The listing builds one solid part. Answer for the finished solid, in the listing's coordinates (mm). A direction names the side the tool comes from. Coordinates: 2 decimals unless noted, no trailing zeros. Order: outer loops, then holes, each group sorted by start corner. A loop starts at its lowest first (then second) coordinate and runs counter-clockwise, first axis right, second up. Notation, with made-up numbers: (-3, 74.5) - (13, 74.5) arc R32 cw to (13, 112.5) - close; hole circle Ø1 at (87.25, 50). An arc over 180 degrees is marked (long way). Use a Markdown table: item, result. Add a question column.
Item 1: The part is cut by section A-A, the plane z = 62. State how many separate pieces and enclosed holes the cut face has, then the cut area to 3 significant figures.
Item 2: Find the intervals of material crossed by line 1 along X through (y, z) = (-29.5, 34); line 2 along Y through (x, z) = (0, 8); line 3 along Y through (x, z) = (0, 41), in increasing order.
Item 3: The part is cut by section B-B, the plane x = 0. Give the vertices of the cut face in (y, z), then the cut area to 3 significant figures.
Item 4: For faces 5 (the cylindrical face through (13.887, -10.648, 4.93)), 6 (the cylindrical face through (23.334, 20.721, 16.661)), 7 (the flat face through (32.5, 0, 33)), determine the directions among +Z, -Z, +X, -X, +Y, -Y from which every point of the face is accessible in a straight line to the end or side of a thin tool.
Item 5: Flat-ended cylindrical pins translate along their axes: P1, Ø10, axis at y = 28, z = 36.5, coming from the +X side; P2, Ø1.5, axis at y = 1, z = 34.5, coming from the -X side; P3, Ø1.5, axis at x = 19.5, y = -22, coming from the -Z side; P4, Ø20, axis at x = 31, y = -34, coming from the +Z side. Find the tip coordinate at first contact, or state that the pin passes through.
Item 6: The part is cut by section C-C, the plane z = 33.5. Give the vertices of the cut face in (x, y), then the cut area to 3 significant figures.
Item 7: The mould has two halves that part along Y. Classify faces 1 (the flat face through (-32, 32, 60)), 2 (the flat face through (-41, -18, 70)), 3 (the cylindrical face through (46.187, -19.15, 34.51)), 4 (the flat face through (36.92, -25.85, 65.07)): released by +Y, released by -Y, zero draft, split by the parting line, or undercut.
from build123d import *

# Parameters (mm, degrees)
CROQUIS1_R              = 50
CROQUIS1_R_2            = 15.5
SALIENTE_EXTRUIR1_DEPTH = 70
CROQUIS2_R              = 40
CORTAR_EXTRUIR1_DEPTH   = 32
CROQUIS3_R              = 17.5
CORTAR_EXTRUIR2_DEPTH   = 10
CROQUIS4_R              = 40
CROQUIS4_R_2            = 15.5
CORTAR_EXTRUIR3_DEPTH   = 10
CROQUIS5_R              = 2
CORTAR_EXTRUIR4_DEPTH   = 83.24354078
CROQUIS6_R              = 5
CORTAR_EXTRUIR5_DEPTH   = 5
CORTAR_EXTRUIR6_DEPTH   = 10


with BuildPart() as part:
    # Croquis1 → Saliente-Extruir1 (new body)
    with BuildSketch(Plane.XY):
        Circle(CROQUIS1_R)
        Circle(CROQUIS1_R_2, mode=Mode.SUBTRACT)
    extrude(amount=SALIENTE_EXTRUIR1_DEPTH)

    # Croquis2 → Cortar-Extruir1 (cut)
    with BuildSketch(Plane.XY.offset(70)):
        Circle(CROQUIS2_R)
    extrude(amount=-CORTAR_EXTRUIR1_DEPTH, mode=Mode.SUBTRACT)

    # Croquis3 → Cortar-Extruir2 (cut)
    with BuildSketch(Plane(origin=(0, 0, 0), x_dir=(-1, 0, 0), z_dir=(0, 0, -1))):
        Circle(CROQUIS3_R)
    extrude(amount=-CORTAR_EXTRUIR2_DEPTH, mode=Mode.SUBTRACT)

    # Croquis4 → Cortar-Extruir3 (cut)
    # profile 1 of 2: a face of its own
    with BuildSketch(Plane.XY.offset(38)):
        Circle(CROQUIS4_R)
        with BuildLine():
            Line((-2.5, 27.386127875), (-2.5, 32.5))
            Line((-2.5, 32.5), (2.5, 32.5))
            Line((2.5, 32.5), (2.5, 27.386127875))
            ThreePointArc((2.5, 27.386127875), (19.445436483, 19.445436483), (27.386127875, 2.5))
            Line((27.386127875, 2.5), (32.5, 2.5))
            Line((32.5, 2.5), (32.5, -2.5))
            Line((32.5, -2.5), (27.386127875, -2.5))
            ThreePointArc((27.386127875, -2.5), (19.445436483, -19.445436483), (2.5, -27.386127875))
            Line((2.5, -27.386127875), (2.5, -32.5))
            Line((2.5, -32.5), (-2.5, -32.5))
            Line((-2.5, -32.5), (-2.5, -27.386127875))
            ThreePointArc((-2.5, -27.386127875), (-19.445436483, -19.445436483), (-27.386127875, -2.5))
            Line((-27.386127875, -2.5), (-32.5, -2.5))
            Line((-32.5, -2.5), (-32.5, 2.5))
            Line((-32.5, 2.5), (-27.386127875, 2.5))
            ThreePointArc((-27.386127875, 2.5), (-19.445436483, 19.445436483), (-2.5, 27.386127875))
        make_face(mode=Mode.SUBTRACT)
    # profile 2 of 2: a face of its own
    with BuildSketch(Plane.XY.offset(38)):
        with BuildLine():
            Line((-2.5, 22.5), (-2.5, 27.386127875))
            ThreePointArc((-2.5, 27.386127875), (-19.445436483, 19.445436483), (-27.386127875, 2.5))
            Line((-27.386127875, 2.5), (-22.5, 2.5))
            Line((-22.5, 2.5), (-22.5, -2.5))
            Line((-22.5, -2.5), (-27.386127875, -2.5))
            ThreePointArc((-27.386127875, -2.5), (-19.445436483, -19.445436483), (-2.5, -27.386127875))
            Line((-2.5, -27.386127875), (-2.5, -22.5))
            Line((-2.5, -22.5), (2.5, -22.5))
            Line((2.5, -22.5), (2.5, -27.386127875))
            ThreePointArc((2.5, -27.386127875), (19.445436483, -19.445436483), (27.386127875, -2.5))
            Line((27.386127875, -2.5), (22.5, -2.5))
            Line((22.5, -2.5), (22.5, 2.5))
            Line((22.5, 2.5), (27.386127875, 2.5))
            ThreePointArc((27.386127875, 2.5), (19.445436483, 19.445436483), (2.5, 27.386127875))
            Line((2.5, 27.386127875), (2.5, 22.5))
            Line((2.5, 22.5), (-2.5, 22.5))
        make_face()
        with Locations(Location((0, 0, 0), (0, 0, 180))):
            Circle(CROQUIS4_R_2, mode=Mode.SUBTRACT)
    extrude(amount=-CORTAR_EXTRUIR3_DEPTH, mode=Mode.SUBTRACT)

    # Croquis5 → Cortar-Extruir4 (cut, through all)
    with BuildSketch(Plane.XY.offset(28)):
        with Locations((21.486974797, 21.486974797)):
            Circle(CROQUIS5_R)
        with Locations((21.486974797, -21.486974797)):
            Circle(CROQUIS5_R)
        with Locations((-21.486974797, -21.486974797)):
            Circle(CROQUIS5_R)
        with Locations((-21.486974797, 21.486974797)):
            Circle(CROQUIS5_R)
    extrude(amount=-CORTAR_EXTRUIR4_DEPTH, mode=Mode.SUBTRACT)

    # Croquis6 → Cortar-Extruir5 (cut)
    with BuildSketch(Plane(origin=(0, 0, 0), x_dir=(-1, 0, 0), z_dir=(0, 0, -1))):
        with Locations((-21.486974797, 21.486974797)):
            Circle(CROQUIS6_R)
        with Locations((21.486974797, 21.486974797)):
            Circle(CROQUIS6_R)
        with Locations((21.486974797, -21.486974797)):
            Circle(CROQUIS6_R)
        with Locations((-21.486974797, -21.486974797)):
            Circle(CROQUIS6_R)
    extrude(amount=-CORTAR_EXTRUIR5_DEPTH, mode=Mode.SUBTRACT)

    # Croquis7 → Cortar-Extruir6 (cut)
    with BuildSketch(Plane.XY.offset(70)):
        with BuildLine():
            ThreePointArc((-6.945927107, 39.39231012), (-3.48622971, 39.847787924), (0, 40))
            Line((0, 40), (0, 50))
            ThreePointArc((0, 50), (-4.357787137, 49.809734905), (-8.682408883, 49.240387651))
            Line((-8.682408883, 49.240387651), (-6.945927107, 39.39231012))
        make_face()
        with BuildLine():
            Line((0, 50), (0, 40))
            ThreePointArc((0, 40), (3.48622971, 39.847787924), (6.945927107, 39.39231012))
            Line((6.945927107, 39.39231012), (8.682408883, 49.240387651))
            ThreePointArc((8.682408883, 49.240387651), (4.357787137, 49.809734905), (0, 50))
        make_face()
        with BuildLine():
            ThreePointArc((22.943057454, 32.766081772), (28.284271247, 28.284271247), (32.766081772, 22.943057454))
            Line((32.766081772, 22.943057454), (40.957602214, 28.678821818))
            ThreePointArc((40.957602214, 28.678821818), (35.355339059, 35.355339059), (28.678821818, 40.957602214))
            Line((28.678821818, 40.957602214), (22.943057454, 32.766081772))
        make_face()
        with BuildLine():
            ThreePointArc((40, 0), (39.847787924, -3.48622971), (39.39231012, -6.945927107))
            Line((39.39231012, -6.945927107), (49.240387651, -8.682408883))
            ThreePointArc((49.240387651, -8.682408883), (49.809734905, -4.357787137), (50, 0))
            ThreePointArc((50, 0), (49.809734905, 4.357787137), (49.240387651, 8.682408883))
            Line((49.240387651, 8.682408883), (39.39231012, 6.945927107))
            ThreePointArc((39.39231012, 6.945927107), (39.847787924, 3.48622971), (40, 0))
        make_face()
        with BuildLine():
            ThreePointArc((32.766081772, -22.943057454), (28.284271247, -28.284271247), (22.943057454, -32.766081772))
            Line((22.943057454, -32.766081772), (28.678821818, -40.957602214))
            ThreePointArc((28.678821818, -40.957602214), (35.355339059, -35.355339059), (40.957602214, -28.678821818))
            Line((40.957602214, -28.678821818), (32.766081772, -22.943057454))
        make_face()
        with BuildLine():
            ThreePointArc((-32.766081772, 22.943057454), (-28.284271247, 28.284271247), (-22.943057454, 32.766081772))
            Line((-22.943057454, 32.766081772), (-28.678821818, 40.957602214))
            ThreePointArc((-28.678821818, 40.957602214), (-35.355339059, 35.355339059), (-40.957602214, 28.678821818))
            Line((-40.957602214, 28.678821818), (-32.766081772, 22.943057454))
        make_face()
        with BuildLine():
            ThreePointArc((-39.39231012, -6.945927107), (-40, 0), (-39.39231012, 6.945927107))
            Line((-39.39231012, 6.945927107), (-49.240387651, 8.682408883))
            ThreePointArc((-49.240387651, 8.682408883), (-50, 0), (-49.240387651, -8.682408883))
            Line((-49.240387651, -8.682408883), (-39.39231012, -6.945927107))
        make_face()
        with BuildLine():
            ThreePointArc((-22.943057454, -32.766081772), (-28.284271247, -28.284271247), (-32.766081772, -22.943057454))
            Line((-32.766081772, -22.943057454), (-40.957602214, -28.678821818))
            ThreePointArc((-40.957602214, -28.678821818), (-35.355339059, -35.355339059), (-28.678821818, -40.957602214))
            Line((-28.678821818, -40.957602214), (-22.943057454, -32.766081772))
        make_face()
        with BuildLine():
            ThreePointArc((6.945927107, -39.39231012), (0, -40), (-6.945927107, -39.39231012))
            Line((-6.945927107, -39.39231012), (-8.682408883, -49.240387651))
            ThreePointArc((-8.682408883, -49.240387651), (0, -50), (8.682408883, -49.240387651))
            Line((8.682408883, -49.240387651), (6.945927107, -39.39231012))
        make_face()
    extrude(amount=-CORTAR_EXTRUIR6_DEPTH, mode=Mode.SUBTRACT)


solid = part.part
Solution:
| question | item | result |
|---|---|---|
| 1 | separate pieces | 8 |
| 1 | enclosed holes | 0 |
| 1 | area | 1,570 mm2 |
| 2 | line 1 | x = -40.37 to -27.01, -2.5 to 2.5, 27.01 to 40.37 |
| 2 | line 2 | y = -50 to -17.5, 17.5 to 50 |
| 2 | line 3 | y = -50 to -40, 40 to 50 |
| 3 | outline | (-50, 0) - (-17.5, 0) - (-17.5, 10) - (-15.5, 10) - (-15.5, 28) - (-22.5, 28) - (-22.5, 38) - (-32.5, 38) - (-32.5, 28) - (-40, 28) - (-40, 60) - (-50, 60) - close; (15.5, 10) - (17.5, 10) - (17.5, 0) - (50, 0) - (50, 60) - (40, 60) - (40, 28) - (32.5, 28) - (32.5, 38) - (22.5, 38) - (22.5, 28) - (15.5, 28) - close |
| 3 | area | 2,730 mm2 |
| 4 | face 5 | -Z |
| 4 | face 6 | +Z, -Z |
| 4 | face 7 | +Z |
| 5 | P1 | stops at x = 44.4 |
| 5 | P2 | stops at x = -50 |
| 5 | P3 | stops at z = 5 |
| 5 | P4 | stops at z = 70 |
| 6 | outline | circle Ø100 at (0, 0); (-32.5, -2.5) - (-22.5, -2.5) - (-22.5, 2.5) - (-32.5, 2.5) - close; (-2.5, -32.5) - (2.5, -32.5) - (2.5, -22.5) - (-2.5, -22.5) - close; (-2.5, 22.5) - (2.5, 22.5) - (2.5, 32.5) - (-2.5, 32.5) - close; (22.5, -2.5) - (32.5, -2.5) - (32.5, 2.5) - (22.5, 2.5) - close; hole circle Ø80 at (0, 0) |
| 6 | area | 3,030 mm2 |
| 7 | face 1 | undercut |
| 7 | face 2 | zero draft |
| 7 | face 3 | split by the parting line |
| 7 | face 4 | released by -Y |
